```python
from build123d import *

# Parameters (mm, degrees)
F0_R     = 7.5
F0_R_2   = 5
F0_R_3   = 12.5
F0_R_4   = 10.5
F1_DEPTH = 1.5
F2_DEPTH = 4
F3_DEPTH = 16
F4_SIZE  = 1


with BuildPart() as f1:
    # F0 (on Top) → F1 (new body)
    with BuildSketch(Plane.XY):
        Circle(F0_R)
        Circle(F0_R_2, mode=Mode.SUBTRACT)
        Circle(F0_R_3)
        Circle(F0_R_4, mode=Mode.SUBTRACT)
        Circle(F0_R_4)
        Circle(F0_R, mode=Mode.SUBTRACT)
    extrude(amount=F1_DEPTH)

    # F0 (on Top) → F2 (join)
    with BuildSketch(Plane.XY):
        Circle(F0_R)
        Circle(F0_R_2, mode=Mode.SUBTRACT)
        Circle(F0_R_4)
        Circle(F0_R, mode=Mode.SUBTRACT)
    extrude(amount=F2_DEPTH)

    # F0 (on Top) → F3 (join)
    with BuildSketch(Plane.XY):
        Circle(F0_R)
        Circle(F0_R_2, mode=Mode.SUBTRACT)
    extrude(amount=F3_DEPTH)

    # F4
    f4_edges = [f1.edges().sort_by_distance(p)[0] for p in [
        (-7.5, 0, 16),
        (-7.5, 0, 4),
    ]]
    chamfer(f4_edges, length=F4_SIZE)


solid = f1.part
```
For this review, take the finished solid that the model builds, in its own axes (mm). A direction names the side the tool comes from. Round coordinates to 2 decimals unless told otherwise and drop trailing zeros. Write each loop counter-clockwise with the first axis right and the second up, starting at its lowest first coordinate (ties: lowest second). Pieces come first, ordered by that corner, then holes. Notation, with made-up numbers: M 88.25,21 L 104.25,21 A19 cw 104.25,37 Z; hole C 33,14.25 d5. An arc over 180 degrees is marked long. One line per item, written item: value. Start each with the question number.
(1) The part is to be moulded in two halves that separate along X. For faces 3 (the cylindrical face through (11.923, 3.755, 0.74)), 4 (the cylindrical face through (-1.08, -4.88, 7.89)), 5 (the flat face through (2, -5, 16)), say which applies: released by +X, released by -X, zero draft, split by the parting line, or undercut.
(2) Wall thickness on line 1 (Y direction, x = 0, z = 5.75); line 2 (Y direction, x = 0, z = 3.5); line 3 (Z direction, x = -6.5, y = 0.25): over which ranges is each line inside the solid? List them lowest first.
(3) We need section C-C (z = 11). Give the boundary of the cut face in (x, y), and give its area (3 significant figures).
(4) Insertion check: pin 1 (4 mm diameter, centred on x = 6.5, z = 13, fed in from +Y); pin 2 (8 mm diameter, centred on x = 0.5, z = 6.5, fed in from -Y); pin 3 (8 mm diameter, centred on y = 2.5, z = 13.5, fed in from +X). Each pin has a flat end and moves straight along its axis. Give the tip position at first contact, or say it passes through.
(5) We need section A-A (x = 0). Give the boundary of the cut face in (y, z).
(6) Machinability: for faces 1 (the flat face through (-0.2, -5.4, 0)), 2 (the cylindrical face through (10, 3.2, 2.7)), which of the approach directions +Z, -Z, +X, -X, +Y, -Y give a long, thin tool a straight path to every point of the face, cutting with its end or side? Answer none if there is none.
(7) We need section D-D (y = 11.25). Give the boundary of the cut face in (x, z), and give its area (3 significant figures).
Result:
1. face 3: split by the parting line
1. face 4: undercut
1. face 5: zero draft
2. line 1: -7.5 to -5, 5 to 7.5
2. line 2: -10.5 to -5, 5 to 10.5
2. line 3: 0 to 16
3. outline: C 0,0 d15; hole C 0,0 d10
3. area: 98.2 mm²
4. pin 1: y = 6
4. pin 2: y = -10.5
4. pin 3: x = 7.5
5. outline: M -12.5,0 L -5,0 L -5,16 L -6.5,16 L -7.5,15 L -7.5,5 L -8.5,4 L -10.5,4 L -10.5,1.5 L -12.5,1.5 Z; M 5,0 L 12.5,0 L 12.5,1.5 L 10.5,1.5 L 10.5,4 L 8.5,4 L 7.5,5 L 7.5,15 L 6.5,16 L 5,16 Z
6. face 1: -Z, +X, -X, +Y, -Y
6. face 2: +Z
7. outline: M -5.45,0 L 5.45,0 L 5.45,1.5 L -5.45,1.5 Z
7. area: 16.3 mm²
